Check sheet for the modelled part. Datum: model origin and axes. Units: mm. A direction names the side the tool comes from. Coordinates: 2 decimals unless noted, no trailing zeros. Loops run counter-clockwise (first coordinate to the right, second up) from the corner with the lowest first, then second, coordinate; pieces in that order, holes last. Notation, with made-up numbers: (66, 84) -> (102, 84) arc R22 cw to (102, 123) -> close; hole circle Ø6 at (73, 70). An arc over 180 degrees is marked (long way). Use one line per item in the form item = value.
from build123d import *

# Parameters (mm, degrees)
F1_DEPTH = 60
F2_R     = 6.25
F3_DEPTH = 2
F4_DEPTH = 2
F5_R     = 1.5
F6_DEPTH = 2
F7_R     = 1.5
F8_DEPTH = 2


with BuildPart() as f1:
    # F0 (on Top) → F1 (new body)
    with BuildSketch(Plane.XY):
        Polygon((0, 2), (0, 0), (7.0000001118, 0), (7.0000001118, 34.142), (30, 34.142), (44.142, 19.9997287538), (44.142, 0), (54.142, 0), (54.142, 2), (46.142, 2), (46.142, 20.8281446432), (30.8284383602, 36.142), (5.0000001118, 36.142), (5.0000001118, 2), align=None)
    extrude(amount=F1_DEPTH)

    # F2 (on face) → F3 (cut)
    with BuildSketch(Plane(origin=(33.4855148215, 33.4848725755, 0), x_dir=(-0.7071, 0.7071135623, 0), z_dir=(0.7071135623, 0.7071, 0))):
        with Locations((-7.1303164004, 40)):
            Circle(F2_R)
    extrude(amount=-F3_DEPTH, mode=Mode.SUBTRACT)

    # F2 (on face) → F4 (cut)
    with BuildSketch(Plane(origin=(33.4855148215, 33.4848725755, 0), x_dir=(-0.7071, 0.7071135623, 0), z_dir=(0.7071135623, 0.7071, 0))):
        with Locations((-7.0707175203, 20)):
            Circle(F2_R)
    extrude(amount=-F4_DEPTH, mode=Mode.SUBTRACT)

    # F5 (on face) → F6 (cut)
    with BuildSketch(Plane(origin=(0, 2, 0), x_dir=(-1, 0, 0), z_dir=(0, 1, 0))):
        with Locations((-50.142, 45)):
            Circle(F5_R)
        with Locations((-50.142, 15)):
            Circle(F5_R)
    extrude(amount=-F6_DEPTH, mode=Mode.SUBTRACT)

    # F7 (on face) → F8 (cut)
    with BuildSketch(Plane(origin=(0, 2, 0), x_dir=(-1, 0, 0), z_dir=(0, 1, 0))):
        with Locations((-2.5000000559, 15)):
            Circle(F7_R)
        with Locations((-2.5000000559, 45)):
            Circle(F7_R)
    extrude(amount=-F8_DEPTH, mode=Mode.SUBTRACT)


solid = f1.part
(1) Section check D-D, the plane z = 38. Record the boundary of the cut face in (x, y), plus the area to 3 significant figures.
Established:
outline = (0, 0) -> (7, 0) -> (7, 34.14) -> (30, 34.14) -> (32.93, 31.22) -> (34.34, 32.63) -> (30.83, 36.14) -> (5, 36.14) -> (5, 2) -> (0, 2) -> close; (41.3, 22.84) -> (44.14, 20) -> (44.14, 0) -> (54.14, 0) -> (54.14, 2) -> (46.14, 2) -> (46.14, 20.83) -> (42.71, 24.26) -> close
area = 204 mm²
(2) Tool access check on faces 5 (the flat face through (46.142, 11, 30)), 6 (the flat face through (5, 19, 30)), 7 (the flat face through (18, 34.142, 30)). Record the directions out of +Z, -Z, +X, -X, +Y, -Y that give a thin tool (end or side, any length) a straight path to the whole face; none if there is none.
Established:
face_5 = +Z, -Z, +X, +Y
face_6 = +Z, -Z, -X, +Y
face_7 = +Z, -Z, -Y
(3) Go/stop test with flat-tipped pins: P1, Ø5, axis at y = 25, z = 28.5, coming from the -X side; P2, Ø10, axis at x = 48, y = 8, coming from the +Z side; P3, Ø7, axis at x = 23.5, z = 22.5, coming from the -Y side; P4, Ø2.5, axis at x = 2.5, z = 45, coming from the +Y side. Record where each tip stops, or that it passes through.
Established:
P1 = 5
P2 = 60
P3 = 34.14
P4 = through
(4) Section check B-B, the plane y = 7.5. Record the boundary of the cut face in (x, z), plus the area to 3 significant figures.
Established:
outline = (5, 0) -> (7, 0) -> (7, 60) -> (5, 60) -> close; (44.14, 0) -> (46.14, 0) -> (46.14, 60) -> (44.14, 60) -> close
area = 240 mm²
(5) Scan lines: line 1 along Z through (x, y) = (2.5, 1.1); line 2 along X through (y, z) = (6, 39); line 3 along Y through (x, z) = (20, 14). Record each from-to range of solid material in increasing order.
Established:
line_1 = 0 to 13.5, 16.5 to 43.5, 46.5 to 60
line_2 = 5 to 7, 44.14 to 46.14
line_3 = 34.14 to 36.14
(6) Section check A-A, the plane x = 2.5. Record the boundary of the cut face in (y, z), plus the area to 3 significant figures.
Established:
outline = (0, 0) -> (2, 0) -> (2, 13.5) -> (0, 13.5) -> close; (0, 16.5) -> (2, 16.5) -> (2, 43.5) -> (0, 43.5) -> close; (0, 46.5) -> (2, 46.5) -> (2, 60) -> (0, 60) -> close
area = 108 mm²
(7) Mould release check, pull along Z, two halves, no side actions. Record for faces 1 (the flat face through (50, 2, 30)), 2 (the cylindrical face through (3.61, 1.01, 16.01)), 3 (the cylindrical face through (48.71, 1.01, 15.45)), 4 (the flat face through (33, 32, 60)): +Z half, -Z half, draft (parallel to the pull), parting line (faces both ways), or undercut.
Established:
face_1 = draft
face_2 = undercut
face_3 = undercut
face_4 = +Z half
(8) Section check C-C, the plane z = 45. Record the boundary of the cut face in (x, y), plus the area to 3 significant figures.
Established:
outline = (0, 0) -> (1, 0) -> (1, 2) -> (0, 2) -> close; (4, 0) -> (7, 0) -> (7, 34.14) -> (30, 34.14) -> (34.46, 29.68) -> (35.88, 31.09) -> (30.83, 36.14) -> (5, 36.14) -> (5, 2) -> (4, 2) -> close; (39.76, 24.38) -> (44.14, 20) -> (44.14, 0) -> (48.64, 0) -> (48.64, 2) -> (46.14, 2) -> (46.14, 20.83) -> (41.18, 25.79) -> close; (51.64, 0) -> (54.14, 0) -> (54.14, 2) -> (51.64, 2) -> close
area = 201 mm²
